Design review of the part built by this model. Coordinates are the model's own, in mm. A direction names the side the tool comes from. Coordinates: 2 decimals unless noted, no trailing zeros. Loops run counter-clockwise (first coordinate to the right, second up) from the corner with the lowest first, then second, coordinate; pieces in that order, holes last. Notation, with made-up numbers: (-7.5, 0.5) -> (3.5, 0.5) arc R21 ccw to (3.5, 5.5) -> close; hole circle Ø10 at (46, -20.5). An arc over 180 degrees is marked (long way). Answer in a Markdown table with one row per item.
```python
from build123d import *

# Parameters (mm, degrees)
ENL_V_MAT_EXTRU_1_DEPTH = 8


with BuildPart() as part:
    # Esquisse1 → Révolution1 (revolve)
    with BuildSketch(Plane.XY, mode=Mode.PRIVATE) as r_volution1_sk:
        Polygon((0, 0), (0, 6.7), (0.3, 7), (3.7, 7), (4, 6.7), (4, 4.5), (4.5, 4.5), (4.5, 5), (12.1, 5), (12.4, 4.7), (12.4, 0), align=None)
    revolve(r_volution1_sk.sketch.rotate(Axis((-14.206779661, 0, 0), (1, 0, 0)), 90), axis=Axis((-14.206779661, 0, 0), (1, 0, 0)))

    # Esquisse2 → Enlèv. mat.-Extru.1 (cut)
    with BuildSketch(Plane.ZY):
        Polygon((-1.443375673, 2.5), (1.443375673, 2.5), (2.886751346, 0), (1.443375673, -2.5), (-1.443375673, -2.5), (-2.886751346, 0), align=None)
    extrude(amount=-ENL_V_MAT_EXTRU_1_DEPTH, mode=Mode.SUBTRACT)


solid = part.part
```
(1) For pin 1 (1 mm diameter, centred on x = 6, y = 4.5, fed in from -Z); pin 2 (6 mm diameter, centred on x = 7.5, y = 5, fed in from -Z); pin 3 (4 mm diameter, centred on x = 2.5, z = -5, fed in from -Y), all flat-tipped, find the tip position at first contact; note any pin that passes through.
Evaluation:
| item | result |
|---|---|
| pin 1 | stops at z = -3 |
| pin 2 | stops at z = -4.58 |
| pin 3 | stops at y = -6.32 |
(2) To check wall thickness, follow probe 1 along Y at (x, z) = (1, 0.25); probe 2 along Y at (x, z) = (6.5, 0.75); probe 3 along Z at (x, y) = (2.25, 0.5). State the ranges of each line that lie inside material, in increasing order.
Evaluation:
| item | result |
|---|---|
| probe 1 | y = -7 to -2.5, 2.5 to 7 |
| probe 2 | y = -4.94 to -2.5, 2.5 to 4.94 |
| probe 3 | z = -6.98 to -2.6, 2.6 to 6.98 |
(3) Take a section at B-B on z = 0. Give the boundary of the cut face in (x, y).
Evaluation:
| item | result |
|---|---|
| outline | (0, -6.7) -> (0.3, -7) -> (3.7, -7) -> (4, -6.7) -> (4, -4.5) -> (4.5, -4.5) -> (4.5, -5) -> (12.1, -5) -> (12.4, -4.7) -> (12.4, 4.7) -> (12.1, 5) -> (4.5, 5) -> (4.5, 4.5) -> (4, 4.5) -> (4, 6.7) -> (3.7, 7) -> (0.3, 7) -> (0, 6.7) -> (0, 2.5) -> (8, 2.5) -> (8, -2.5) -> (0, -2.5) -> close |
(4) Draft analysis for pull direction Z (two halves, no side actions). For faces 4 (the flat face through (0, 3, 0)), 5 (the cylindrical face through (8, 0, -5)), 6 (the flat face through (8, 0, 0)), 7 (the flat face through (3.944, 1.233, -2.175)), state which applies: pulls with the +Z half, pulls with the -Z half, needs draft (parallel to the pull), parting line crosses it, or undercut.
Evaluation:
| item | result |
|---|---|
| face 4 | needs draft |
| face 5 | parting line crosses it |
| face 6 | undercut |
| face 7 | undercut |
(5) Tool access review of faces 1 (the flat face through (4, -2.5, 0)), 2 (the cylindrical face through (4.25, -3.04, -3.32)), 3 (the flat face through (12.4, 0, 0)): name each direction out of +Z, -Z, +X, -X, +Y, -Y from which nothing blocks a thin tool from reaching the whole face with its end or side.
Evaluation:
| item | result |
|---|---|
| face 1 | -X |
| face 2 | none |
| face 3 | +Z, -Z, +X, +Y, -Y |
(6) Take a section at C-C on x = 5.5. Give the boundary of the cut face in (y, z).
Evaluation:
| item | result |
|---|---|
| outline | circle Ø10 at (0, 0); hole (-2.5, -1.44) -> (0, -2.89) -> (2.5, -1.44) -> (2.5, 1.44) -> (0, 2.89) -> (-2.5, 1.44) -> close |
(7) Take a section at A-A on x = 3. Give the boundary of the cut face in (y, z), and give its area (3 significant figures).
Evaluation:
| item | result |
|---|---|
| outline | circle Ø14 at (0, 0); hole (-2.5, -1.44) -> (0, -2.89) -> (2.5, -1.44) -> (2.5, 1.44) -> (0, 2.89) -> (-2.5, 1.44) -> close |
| area | 132 mm² |
